Geometry: final body of the model. Coordinates: model frame, mm. A direction names the side the tool comes from. Round coordinates to 2 decimals unless told otherwise and drop trailing zeros. Loops run counter-clockwise (first coordinate to the right, second up) from the corner with the lowest first, then second, coordinate; pieces in that order, holes last. Notation, with made-up numbers: (14.25, 26) - (64.25, 26) arc R12 ccw to (64.25, 34) - close; hole circle Ø11 at (48.25, 60.5). An arc over 180 degrees is marked (long way). Write item = value, one per line. Start each with the question number.
Item 1: Section B-B (y = 38). Return loops of the section in (x, z), plus the area to 3 significant figures.
Item 2: Access query for faces 1 (the flat face through (-42.5, 33, 2)), 2 (the flat face through (0, 4, 0)), 3 (the flat face through (-9.5, 33, 3)), 4 (the flat face through (-22, 46, -15)), 5 (the cylindrical face through (-11.004, 33.994, -15.45)). Directions: +Z, -Z, +X, -X, +Y, -Y. A direction counts if a zero-diameter tool reaches every point of the face in a straight line with its end or side. Return the directions, or none.
Item 3: Draft query along Z for faces 6 (the flat face through (-26, 14.235, 2)), 7 (the flat face through (-1.97, 3.48, 12.4)), 8 (the cylindrical face through (-26.16, 55.73, -15.45)), 9 (the cylindrical face through (-0.99, 9.64, 12.96)). Return one class per face: pulls with the +Z half, pulls with the -Z half, needs draft (parallel to the pull), parting line crosses it, or undercut.
Item 4: Section C-C (z = -9). Return loops of the section in (x, y).
Item 5: First-contact query: pin 1 (8 mm diameter, centred on y = 0, z = 0, fed in from -X); pin 2 (1.1 mm diameter, centred on x = -27, y = 15, fed in from -Z); pin 3 (2 mm diameter, centred on x = -51.5, y = 15, fed in from -Z); pin 4 (21 mm diameter, centred on x = -33, z = 5, fed in from -Y). Flat tips, straight axial feed; report the tip coordinate or a pass-through.
Item 6: Section D-D (x = -40.5). Return loops of the section in (y, z).
Item 7: Section A-A (x = -26). Return loops of the section in (y, z).
Item 8: Line query: line 1 (Z direction, x = -26, y = 12.4); line 2 (Y direction, x = -21, z = 13.5); line 3 (Y direction, x = -1, z = 0). Output: solid intervals per line, ascending. Write a range as from..to.
from build123d import *

# Parameters (mm, degrees)
SKETCH_1_R          = 9
SKETCH_1_R_2        = 2.5
EXTRUDE_1_DEPTH     = 4
EXTRUDE_2_DEPTH     = 4
SKETCH_6_W          = 33.754755736
SKETCH_6_H          = 3
EXTRUDE_5_DEPTH     = 52
SKETCH_7_R          = 2.5
EXTRUDE_6_DEPTH     = 4
SKETCH_8_R          = 2.5
EXTRUDE_7_DEPTH     = 8
SKETCH_9_W          = 27
SKETCH_9_H          = 3
EXTRUDE_8_DEPTH     = 40
SKETCH_10_W         = 8
SKETCH_10_H         = 8
CUT_EXTRUDE_1_DEPTH = 40
SKETCH_11_W         = 27
SKETCH_11_H         = 30.754755736
EXTRUDE_9_DEPTH     = 3
SKETCH_12_R         = 35
SKETCH_12_W         = 33
SKETCH_12_H         = 33.754755736
EXTRUDE_10_DEPTH    = 4
SKETCH_13_R         = 2
CUT_EXTRUDE_2_DEPTH = 4
FILLET_1_R          = 5
SKETCH_14_R         = 5
CUT_EXTRUDE_3_DEPTH = 3
CUT_EXTRUDE_4_DEPTH = 2
SKETCH_16_R         = 3.5
CUT_EXTRUDE_5_DEPTH = 6


with BuildPart() as part:
    # 草图1 → 凸台-拉伸1 (new body)
    with BuildSketch(Plane(origin=(0, 0, 0), x_dir=(0, 0, -1), z_dir=(1, 0, 0))):
        Circle(SKETCH_1_R)
        Circle(SKETCH_1_R_2, mode=Mode.SUBTRACT)
    extrude(amount=-EXTRUDE_1_DEPTH)

    # 草图2 → 凸台-拉伸2 (add)
    with BuildSketch(Plane(origin=(0, 0, 0), x_dir=(0, 0, -1), z_dir=(1, 0, 0))):
        with BuildLine():
            Line((-16.878750928, 11.234854176), (-7.794228634, -4.5))
            ThreePointArc((-7.794228634, -4.5), (-2.329371406, 8.693332437), (9, 0))
            ThreePointArc((9, 0), (8.719533008, -2.229292291), (7.895612418, -4.319641714))
            Line((7.895612418, -4.319641714), (16.876004808, 11.234854176))
            Line((16.876004808, 11.234854176), (-16.878750928, 11.234854176))
        make_face()
    extrude(amount=-EXTRUDE_2_DEPTH)

    # 草图6 → 凸台-拉伸5 (add)
    with BuildSketch(Plane(origin=(0, 0, 0), x_dir=(0, 0, -1), z_dir=(1, 0, 0))):
        with Locations((-0.00137306, 12.734854176)):
            Rectangle(SKETCH_6_W, SKETCH_6_H)
    extrude(amount=-EXTRUDE_5_DEPTH)

    # 草图7 → 凸台-拉伸6 (add)
    with BuildSketch(Plane(origin=(-35.5, 0, 0), x_dir=(0, 0, -1), z_dir=(1, 0, 0))):
        with BuildLine():
            Line((-16.878750928, 11.234854176), (-7.794228634, -4.5))
            ThreePointArc((-7.794228634, -4.5), (0.103450209, -8.999405428), (7.895612418, -4.319641714))
            Line((7.895612418, -4.319641714), (16.876004808, 11.234854176))
            Line((16.876004808, 11.234854176), (-16.878750928, 11.234854176))
        make_face()
        Circle(SKETCH_7_R, mode=Mode.SUBTRACT)
    extrude(amount=-EXTRUDE_6_DEPTH)

    # 草图8 → 凸台-拉伸7 (add)
    with BuildSketch(Plane(origin=(-35.5, 0, 0), x_dir=(0, 0, -1), z_dir=(1, 0, 0))):
        Circle(SKETCH_8_R)
    extrude(amount=-EXTRUDE_7_DEPTH)

    # 草图9 → 凸台-拉伸8 (add)
    with BuildSketch(Plane(origin=(0, 14.234854176, 0), x_dir=(1, 0, 0), z_dir=(0, 1, 0))):
        Polygon((-12.5, 16.876004808), (-12.5, 13.876004808), (-12.5, -16.878750928), (-9.5, -16.878750928), (-9.5, 16.876004808), align=None)
        Polygon((-39.5, -16.878750928), (-39.5, 13.876004808), (-39.5, 16.876004808), (-42.5, 16.876004808), (-42.5, -16.878750928), align=None)
        with Locations((-26, 15.376004808)):
            Rectangle(SKETCH_9_W, SKETCH_9_H)
    extrude(amount=EXTRUDE_8_DEPTH)

    # 草图10 → 切除-拉伸1 (cut)
    with BuildSketch(Plane.XY.offset(-13.876004808)):
        with Locations((-26, 46.234854176)):
            Rectangle(SKETCH_10_W, SKETCH_10_H)
    extrude(amount=-CUT_EXTRUDE_1_DEPTH, mode=Mode.SUBTRACT)

    # 草图11 → 凸台-拉伸9 (add)
    with BuildSketch(Plane(origin=(0, 54.234854176, 0), x_dir=(1, 0, 0), z_dir=(0, 1, 0))):
        Polygon((-9.5, -16.878750928), (-9.5, 16.876004808), (-42.5, 16.876004808), (-42.5, -16.878750928), (-39.5, -16.878750928), (-39.5, 13.876004808), (-12.5, 13.876004808), (-12.5, -16.878750928), align=None)
        with Locations((-26, -1.50137306)):
            Rectangle(SKETCH_11_W, SKETCH_11_H)
    extrude(amount=EXTRUDE_9_DEPTH)

    # 草图12 → 凸台-拉伸10 (add)
    with BuildSketch(Plane.XZ.offset(-11.234854176)):
        with Locations((-26, 0.00137306)):
            Circle(SKETCH_12_R)
        with Locations((-26, 0.00137306)):
            Rectangle(SKETCH_12_W, SKETCH_12_H, mode=Mode.SUBTRACT)
    extrude(amount=-EXTRUDE_10_DEPTH)

    # 草图13 → 切除-拉伸2 (cut)
    with BuildSketch(Plane(origin=(0, 15.234854176, 0), x_dir=(1, 0, 0), z_dir=(0, 1, 0))):
        with Locations((-26, -24.878750928)):
            Circle(SKETCH_13_R)
    extrude(amount=-CUT_EXTRUDE_2_DEPTH, mode=Mode.SUBTRACT)

    # 圆角1
    fillet_1_edges = [part.edges().sort_by_distance(p)[0] for p in [
        (-9.5, 57.234854176, 0.00137306),
        (-26, 57.234854176, -16.876004808),
        (-42.5, 57.234854176, 0.00137306),
        (-9.5, 36.234854176, -16.876004808),
        (-42.5, 36.234854176, -16.876004808),
    ]]
    fillet(fillet_1_edges, radius=FILLET_1_R)

    # 草图14 → 切除-拉伸3 (cut)
    with BuildSketch(Plane(origin=(0, 14.234854176, 0), x_dir=(1, 0, 0), z_dir=(0, 1, 0))):
        with Locations((-26, -9.878750928)):
            Circle(SKETCH_14_R)
    extrude(amount=-CUT_EXTRUDE_3_DEPTH, mode=Mode.SUBTRACT)

    # 草图15 → 切除-拉伸4 (cut)
    with BuildSketch(Plane(origin=(0, 0, 0), x_dir=(0, 0, -1), z_dir=(1, 0, 0))):
        with BuildLine():
            ThreePointArc((-3.486194042, -0.310565776), (-2.801542224, 2.097942126), (-0.683036299, 3.432704679))
            Line((-0.683036299, 3.432704679), (-10.750051286, 10.010751226))
            ThreePointArc((-10.750051286, 10.010751226), (-12.980710136, 9.609748083), (-12.708559077, 7.359731144))
            Line((-12.708559077, 7.359731144), (-3.486194042, -0.310565776))
        make_face()
    extrude(amount=-CUT_EXTRUDE_4_DEPTH, mode=Mode.SUBTRACT)

    # 草图16 → 切除-拉伸5 (cut)
    with BuildSketch(Plane(origin=(0, 0, 0), x_dir=(0, 0, -1), z_dir=(1, 0, 0))):
        Circle(SKETCH_16_R)
    extrude(amount=-CUT_EXTRUDE_5_DEPTH, mode=Mode.SUBTRACT)


solid = part.part
Taken from the geometry:
q1.outline = (-42.5, -11.88) arc R5 ccw to (-37.5, -16.88) - (-14.5, -16.88) arc R5 ccw to (-9.5, -11.88) - (-9.5, 16.88) - (-12.5, 16.88) - (-12.5, -13.88) - (-39.5, -13.88) - (-39.5, 16.88) - (-42.5, 16.88) - close
q1.area = 273 mm^2
q2.face_1 = +Z, -Z, -X, +Y
q2.face_2 = +Z, -Z, +X, -Y
q2.face_3 = +Z, -Z, +X, +Y
q2.face_4 = +Z, -Z
q2.face_5 = -Z, +X, +Y
q3.face_6 = undercut
q3.face_7 = pulls with the +Z half
q3.face_8 = pulls with the -Z half
q3.face_9 = undercut
q4.outline = (-59.82, 11.23) - (-39.5, 11.23) - (-39.5, -2.41) - (-35.5, -2.41) - (-35.5, 11.23) - (-4, 11.23) - (-4, -2.41) - (0, -2.41) - (0, 11.23) - (7.82, 11.23) - (7.82, 15.23) - (-9.5, 15.23) - (-9.5, 52.23) arc R5 ccw to (-14.5, 57.23) - (-37.5, 57.23) arc R5 ccw to (-42.5, 52.23) - (-42.5, 15.23) - (-59.82, 15.23) - close; hole (-39.5, 14.23) - (-12.5, 14.23) - (-12.5, 54.23) - (-39.5, 54.23) - close
q5.pin_1 = -43.5
q5.pin_2 = -35
q5.pin_3 = -24.99
q5.pin_4 = -9
q6.outline = circle Ø5 at (0, 0); (11.23, -31.85) - (15.23, -31.85) - (15.23, -15.88) - (52.23, -15.88) arc R4 ccw to (56.23, -11.88) - (56.23, 16.88) - (15.23, 16.88) - (15.23, 31.86) - (11.23, 31.86) - close
q7.outline = (11.23, -35) - (15.23, -35) - (15.23, -16.88) - (42.23, -16.88) - (42.23, -13.88) - (14.23, -13.88) - (14.23, 4.88) - (11.23, 4.88) - close; (11.23, 14.88) - (14.23, 14.88) - (14.23, 16.88) - (15.23, 16.88) - (15.23, 22.88) - (11.23, 22.88) - close; (11.23, 26.88) - (15.23, 26.88) - (15.23, 35) - (11.23, 35) - close; (50.23, -16.88) - (52.23, -16.88) arc R5 ccw to (57.23, -11.88) - (57.23, 16.88) - (54.23, 16.88) - (54.23, -13.88) - (50.23, -13.88) - close
q8.line_1 = -35..4.88, 14.88..22.88, 26.88..35
q8.line_2 = 11.23..14.23, 54.23..57.23
q8.line_3 = -9..-3.5, 3.5..15.23
